Part model, mm, in its own coordinate system. Round coordinates to 2 decimals unless told otherwise and drop trailing zeros. Loops run counter-clockwise (first coordinate to the right, second up) from the corner with the lowest first, then second, coordinate; pieces in that order, holes last.
1) Probe line 1 (Z direction, x = 0, y = 2.1); line 2 (Y direction, x = -27.5, z = -2). List the from-to ranges inside material, lowest first.
2) Band-saw the part on A-A, the plane z = 11. Write the cut outline in (x, y).
3) Band-saw the part on B-B, the plane x = -7. Write the cut outline in (y, z), then the cut area to 3 significant figures.
4) Drop flat-ended pins along their axis: P1, Ø10, axis at x = 11, z = -20, coming from the -Y side; P2, Ø2, axis at y = 2.5, z = 7.5, coming from the -X side; P3, Ø1, axis at x = 21.5, y = 1, coming from the +Z side; P4, Ø23, axis at x = 0, z = 0, coming from the -Y side. Give the stop position or say it passes through.
5) Band-saw the part on D-D, the plane z = -24. Write the cut outline in (x, y).
6) Band-saw the part on C-C, the plane y = 2.5. Write the cut outline in (x, z).
from build123d import *

# Parameters (mm, degrees)
SKETCH1_R                = 19
BOSS_EXTRUDE1_DEPTH      = 3.5
SKETCH2_R                = 30
SKETCH2_R_2              = 19
SKETCH2_R_3              = 2.8
BOSS_EXTRUDE2_DEPTH      = 4
CUT_EXTRUDE1_START       = -10
SKETCH3_R                = 19
CUT_EXTRUDE1_DEPTH       = 10
BOSS_EXTRUDE3_DEPTH      = 2
BOSS_EXTRUDE3_DEPTH_BACK = 4
SKETCH4_R                = 2.9
SKETCH5_R                = 4
BOSS_EXTRUDE4_DEPTH      = 4


with BuildPart() as part:
    # Sketch1 → Boss-Extrude1 (new body)
    with BuildSketch(Plane(origin=(0, 0, 0), x_dir=(1, 0, 0), z_dir=(0, 1, 0))):
        with Locations(Location((0, 0, 0), (0, 0, 270))):
            Circle(SKETCH1_R)
    extrude(amount=BOSS_EXTRUDE1_DEPTH)

    # Sketch2 → Boss-Extrude2 (add)
    with BuildSketch(Plane(origin=(0, 0, 0), x_dir=(1, 0, 0), z_dir=(0, 1, 0))):
        with Locations(Location((0, 0, 0), (0, 0, 270))):
            Circle(SKETCH2_R)
        with Locations(Location((0, 0, 0), (0, 0, 270))):
            Circle(SKETCH2_R_2, mode=Mode.SUBTRACT)
        with Locations(Location((0, 25, 0), (0, 0, 270))):
            Circle(SKETCH2_R_3, mode=Mode.SUBTRACT)
        with Locations(Location((21.650635095, -12.5, 0), (0, 0, 270))):
            Circle(SKETCH2_R_3, mode=Mode.SUBTRACT)
        with Locations(Location((-21.650635095, -12.5, 0), (0, 0, 270))):
            Circle(SKETCH2_R_3, mode=Mode.SUBTRACT)
    extrude(amount=BOSS_EXTRUDE2_DEPTH)

    # Sketch3 → Cut-Extrude1 (cut)
    with BuildSketch(Plane(origin=(0, 3.5, 0), x_dir=(1, 0, 0), z_dir=(0, 1, 0)).offset(CUT_EXTRUDE1_START)):
        with Locations(Location((0, 0, 0), (0, 0, 270))):
            Circle(SKETCH3_R)
    extrude(amount=CUT_EXTRUDE1_DEPTH, mode=Mode.SUBTRACT)

    # Sketch4 → Boss-Extrude3 (add, two sides: drawn at the far end of the back side and taken through both)
    with BuildSketch(Plane.XZ.offset(-BOSS_EXTRUDE3_DEPTH_BACK)):
        with Locations(Location((-21.650635095, 12.5, 0), (0, 0, 270))):
            Circle(SKETCH4_R)
        with Locations(Location((21.650635095, 12.5, 0), (0, 0, 270))):
            Circle(SKETCH4_R)
        with Locations(Location((0, -25, 0), (0, 0, 270))):
            Circle(SKETCH4_R)
    extrude(amount=BOSS_EXTRUDE3_DEPTH + BOSS_EXTRUDE3_DEPTH_BACK)

    # Sketch5 → Boss-Extrude4 (add)
    with BuildSketch(Plane(origin=(0, 4, 0), x_dir=(1, 0, 0), z_dir=(0, 1, 0))):
        with Locations((-27.769349467, 11.35179414)):
            Circle(SKETCH5_R)
        with Locations((23.715616837, 18.373065015)):
            Circle(SKETCH5_R)
        with Locations((4.05373263, -29.724859155)):
            Circle(SKETCH5_R)
    extrude(amount=-BOSS_EXTRUDE4_DEPTH)


solid = part.part
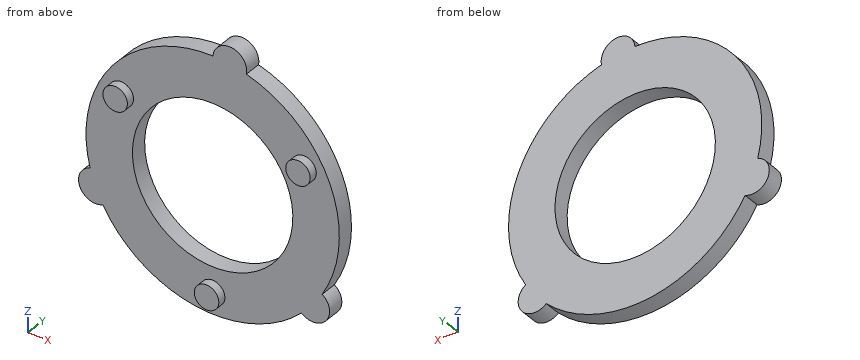
Reported:
1. line 1: z = -30 to -19, 19 to 30
1. line 2: y = 0 to 4
2. outline: (-27.91, 0) - (-24.13, 0) - (-24.13, -2) - (-19.17, -2) - (-19.17, 0) - (-15.49, 0) - (-15.49, 4) - (-27.91, 4) - close; (15.49, 0) - (19.17, 0) - (19.17, -2) - (24.13, -2) - (24.13, 0) - (27.91, 0) - (27.91, 4) - (15.49, 4) - close
3. outline: (0, -29.17) - (4, -29.17) - (4, -17.66) - (0, -17.66) - close; (0, 17.66) - (4, 17.66) - (4, 29.17) - (0, 29.17) - close
3. area: 92.1 mm2
4. P1: stops at y = 0
4. P2: stops at x = -29.29
4. P3: stops at z = 21.42
4. P4: passes through
5. outline: (-18, 0) - (-2.72, 0) - (-2.72, -2) - (2.72, -2) - (2.72, 0) - (18, 0) - (18, 4) - (-18, 4) - close
6. outline: (-29.03, -7.56) arc R4 ccw (long way) to (-26.01, -14.95) arc R30 ccw to (21.06, -21.36) arc R4 ccw (long way) to (25.95, -15.05) arc R30 ccw to (7.97, 28.92) arc R4 ccw (long way) to (0.06, 30) arc R30 ccw to start; hole circle Ø38 at (0, 0)
